```python
from build123d import *

# Parameters (mm, degrees)
SKETCH_3_R           = 9.5
CUT_EXTRUDE_1_DEPTH  = 321.526909947
SKETCH_4_R           = 9.5
CUT_EXTRUDE_2_DEPTH  = 321.526909947
SKETCH_5_R           = 9.5
CUT_EXTRUDE_3_DEPTH  = 321.526909947
SKETCH_6_R           = 9.5
CUT_EXTRUDE_4_DEPTH  = 321.526909947
SKETCH_7_R           = 9.5
CUT_EXTRUDE_5_DEPTH  = 321.526909947
SKETCH_8_R           = 9.5
CUT_EXTRUDE_6_DEPTH  = 321.526909947
SKETCH_9_R           = 9.5
CUT_EXTRUDE_7_DEPTH  = 321.526909947
SKETCH_10_R          = 9.5
CUT_EXTRUDE_8_DEPTH  = 321.526909947
SKETCH_11_R          = 9.5
CUT_EXTRUDE_9_DEPTH  = 321.526909947
SKETCH_12_R          = 9.5
CUT_EXTRUDE_10_DEPTH = 321.526909947
SKETCH_13_R          = 9.5
CUT_EXTRUDE_11_DEPTH = 321.526909947
SKETCH_14_R          = 9.5
CUT_EXTRUDE_12_DEPTH = 321.526909947


with BuildPart() as part:
    # Эскиз1 → Повернуть1 (revolve)
    with BuildSketch(Plane.XY, mode=Mode.PRIVATE) as revolve_1_sk:
        Polygon((0, 0), (265, 0), (265, 127.5), (239, 127.5), (239, 100), (239, 95), (220, 95), (220, 94), (200, 94), (144, 65.5), (70, 65.5), (25, 41), (3, 41), (3, 45), (0, 45), align=None)
    revolve(revolve_1_sk.sketch.rotate(Axis((0, 0, 0), (1, 0, 0)), 90), axis=Axis((0, 0, 0), (1, 0, 0)))

    # Эскиз2 → Вырез-Повернуть1 (revolve, cut)
    with BuildSketch(Plane.XY, mode=Mode.PRIVATE) as cut_revolve_1_sk:
        with BuildLine():
            Line((0, 0), (200, 0))
            Line((200, 0), (200, 55))
            Line((200, 55), (147.669872, 55))
            ThreePointArc((147.669872, 55), (146.273624348, 54.108499061), (146.669872, 52.5))
            Line((146.669872, 52.5), (143.5, 52.5))
            ThreePointArc((143.5, 52.5), (142.75, 52.602347572), (142, 52.5))
            Line((142, 52.5), (90, 52.5))
            ThreePointArc((90, 52.5), (79.13262933, 46.740617582), (70, 38.502577))
            Line((70, 38.502577), (42, 31))
            Line((42, 31), (0, 31))
            Line((0, 31), (0, 0))
        make_face()
    revolve(cut_revolve_1_sk.sketch.rotate(Axis((0, 0, 0), (1, 0, 0)), 90), axis=Axis((0, 0, 0), (1, 0, 0)), mode=Mode.SUBTRACT)

    # Эскиз3 → Вырез-Вытянуть1 (cut, through all)
    with BuildSketch(Plane(origin=(0, 0, 0), x_dir=(0, 0, -1), z_dir=(1, 0, 0))):
        with Locations((0, 113)):
            Circle(SKETCH_3_R)
    extrude(amount=CUT_EXTRUDE_1_DEPTH, mode=Mode.SUBTRACT)

    # Эскиз4 → Вырез-Вытянуть2 (cut, through all)
    with BuildSketch(Plane(origin=(0, 0, 0), x_dir=(0, 0, -1), z_dir=(1, 0, 0))):
        with Locations((-56.5, 97.860870628)):
            Circle(SKETCH_4_R)
    extrude(amount=CUT_EXTRUDE_2_DEPTH, mode=Mode.SUBTRACT)

    # Эскиз5 → Вырез-Вытянуть3 (cut, through all)
    with BuildSketch(Plane(origin=(0, 0, 0), x_dir=(0, 0, -1), z_dir=(1, 0, 0))):
        with Locations((-97.860870628, 56.5)):
            Circle(SKETCH_5_R)
    extrude(amount=CUT_EXTRUDE_3_DEPTH, mode=Mode.SUBTRACT)

    # Эскиз6 → Вырез-Вытянуть4 (cut, through all)
    with BuildSketch(Plane(origin=(0, 0, 0), x_dir=(0, 0, -1), z_dir=(1, 0, 0))):
        with Locations((-113, 0)):
            Circle(SKETCH_6_R)
    extrude(amount=CUT_EXTRUDE_4_DEPTH, mode=Mode.SUBTRACT)

    # Эскиз7 → Вырез-Вытянуть5 (cut, through all)
    with BuildSketch(Plane(origin=(0, 0, 0), x_dir=(0, 0, -1), z_dir=(1, 0, 0))):
        with Locations((-97.860870628, -56.5)):
            Circle(SKETCH_7_R)
    extrude(amount=CUT_EXTRUDE_5_DEPTH, mode=Mode.SUBTRACT)

    # Эскиз8 → Вырез-Вытянуть6 (cut, through all)
    with BuildSketch(Plane(origin=(0, 0, 0), x_dir=(0, 0, -1), z_dir=(1, 0, 0))):
        with Locations((-56.5, -97.860870628)):
            Circle(SKETCH_8_R)
    extrude(amount=CUT_EXTRUDE_6_DEPTH, mode=Mode.SUBTRACT)

    # Эскиз9 → Вырез-Вытянуть7 (cut, through all)
    with BuildSketch(Plane(origin=(0, 0, 0), x_dir=(0, 0, -1), z_dir=(1, 0, 0))):
        with Locations((0, -113)):
            Circle(SKETCH_9_R)
    extrude(amount=CUT_EXTRUDE_7_DEPTH, mode=Mode.SUBTRACT)

    # Эскиз10 → Вырез-Вытянуть8 (cut, through all)
    with BuildSketch(Plane(origin=(0, 0, 0), x_dir=(0, 0, -1), z_dir=(1, 0, 0))):
        with Locations((56.5, -97.860870628)):
            Circle(SKETCH_10_R)
    extrude(amount=CUT_EXTRUDE_8_DEPTH, mode=Mode.SUBTRACT)

    # Эскиз11 → Вырез-Вытянуть9 (cut, through all)
    with BuildSketch(Plane(origin=(0, 0, 0), x_dir=(0, 0, -1), z_dir=(1, 0, 0))):
        with Locations((97.860870628, -56.5)):
            Circle(SKETCH_11_R)
    extrude(amount=CUT_EXTRUDE_9_DEPTH, mode=Mode.SUBTRACT)

    # Эскиз12 → Вырез-Вытянуть10 (cut, through all)
    with BuildSketch(Plane(origin=(0, 0, 0), x_dir=(0, 0, -1), z_dir=(1, 0, 0))):
        with Locations((113, 0)):
            Circle(SKETCH_12_R)
    extrude(amount=CUT_EXTRUDE_10_DEPTH, mode=Mode.SUBTRACT)

    # Эскиз13 → Вырез-Вытянуть11 (cut, through all)
    with BuildSketch(Plane(origin=(0, 0, 0), x_dir=(0, 0, -1), z_dir=(1, 0, 0))):
        with Locations((97.860870628, 56.5)):
            Circle(SKETCH_13_R)
    extrude(amount=CUT_EXTRUDE_11_DEPTH, mode=Mode.SUBTRACT)

    # Эскиз14 → Вырез-Вытянуть12 (cut, through all)
    with BuildSketch(Plane(origin=(0, 0, 0), x_dir=(0, 0, -1), z_dir=(1, 0, 0))):
        with Locations((56.5, 97.860870628)):
            Circle(SKETCH_14_R)
    extrude(amount=CUT_EXTRUDE_12_DEPTH, mode=Mode.SUBTRACT)


solid = part.part
```
For this review, take the finished solid that the model builds, in its own axes (mm). A direction names the side the tool comes from. Round coordinates to 2 decimals unless told otherwise and drop trailing zeros. Loops run counter-clockwise (first coordinate to the right, second up) from the corner with the lowest first, then second, coordinate; pieces in that order, holes last.
Q1. To check wall thickness, follow line 1 along Y through (x, z) = (256, 0); line 2 along Z through (x, y) = (248.5, 96); line 3 along Y through (x, z) = (250, -56.5). State the ranges of each line that lie inside material, in increasing order.
Result sheet:
line 1: y = -127.5 to -122.5, -103.5 to 103.5, 122.5 to 127.5
line 2: z = -83.91 to -65.82, -47.18 to 47.18, 65.82 to 83.91
line 3: y = -114.3 to -107.36, -88.36 to 88.36, 107.36 to 114.3
Q2. Mouldability with a two-part tool opening along X and no side actions: class faces 1 (the face through (3, 40, 10)), 2 (the face through (0, -10.6, 29.4)), 3 (the face through (251.82, -62.28, 105.4)) as +X half, -X half, draft (parallel to the pull), parting line (faces both ways), or undercut.
Result sheet:
face 1: undercut
face 2: -X half
face 3: draft
Q3. Add section C-C on y = 0. Give the number of separate pieces and of enclosed holes in the cut face, plus the area to 3 significant figures.
Result sheet:
separate pieces: 3
enclosed holes: 0
area: 20,300 mm2
Q4. Add section A-A on z = 113. Write out the cut boundary in (x, y).
Result sheet:
outline: (239, -59.05) - (265, -59.05) - (265, -9.5) - (239, -9.5) - close; (239, 9.5) - (265, 9.5) - (265, 59.05) - (239, 59.05) - close
Q5. Machinability: for faces 4 (the face through (229.37, 92.74, -20.59)), 5 (the face through (200, -1, 1)), 6 (the face through (251.818, 103.726, 2.059)), which of the approach directions +Z, -Z, +X, -X, +Y, -Y give a long, thin tool a straight path to every point of the face, cutting with its end or side? Answer none if there is none.
Result sheet:
face 4: -X
face 5: none
face 6: +X, -X
Q6. Insertion check: pin 1 Ø24.5 at (y, z) = (113, 0) entering from -X; pin 2 Ø6 at (x, y) = (226.5, 25.5) entering from +Z; pin 3 Ø8 at (x, z) = (67.5, -71.5) entering from -Y; pin 4 Ø12 at (x, z) = (101, -14.5) entering from -Y. Each pin has a flat end and moves straight along its axis. Give the tip position at first contact, or say it passes through.
Result sheet:
pin 1: stops at x = 239
pin 2: stops at z = 92.3
pin 3: passes through
pin 4: stops at y = -64.95
